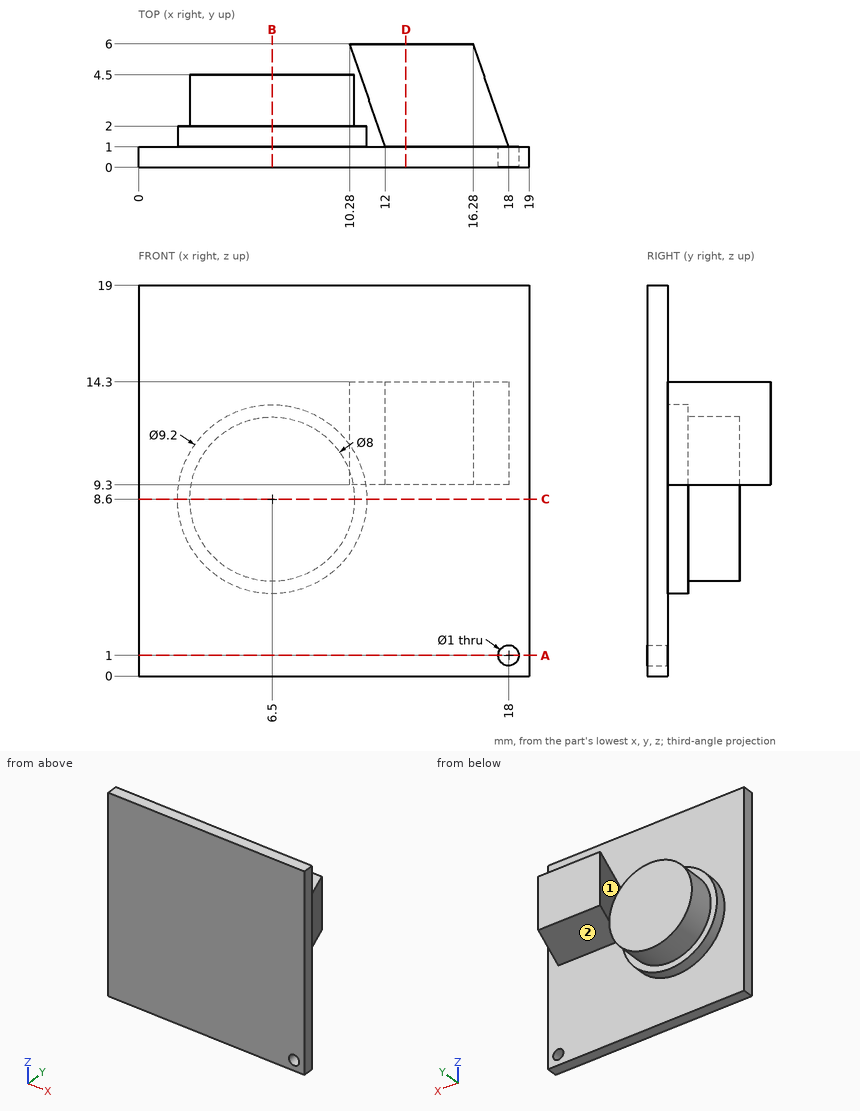
Answer from the drawing. Dimensions are ordinates in mm from the lowest x, y and z of the part. Coordinates: 2 decimals unless noted, no trailing zeros. Write each loop counter-clockwise with the first axis right and the second up, starting at its lowest first coordinate (ties: lowest second). Pieces come first, ordered by that corner, then holes. Notation, with made-up numbers: M 33,-2.75 L 72,-2.75 A10 cw 72,9.25 Z; hole C -28,-32 d11. An arc over 180 degrees is marked long. Use a Markdown table: item, result.
Q1. The part is cut by section D-D, the plane x = 13. Write down the section's boundary in (y, z), then the cut area to 3 significant figures.
Answer block:
| item | result |
|---|---|
| outline | M 0,0 L 1,0 L 1,9.3 L 6,9.3 L 6,14.3 L 1,14.3 L 1,19 L 0,19 Z |
| area | 44.0 mm2 |
Q2. The part is cut by section C-C, the plane z = 8.6. Write down the section's boundary in (x, y), then the cut area to 3 significant figures.
Answer block:
| item | result |
|---|---|
| outline | M 0,0 L 19,0 L 19,1 L 11.1,1 L 11.1,2 L 10.5,2 L 10.5,4.5 L 2.5,4.5 L 2.5,2 L 1.9,2 L 1.9,1 L 0,1 Z |
| area | 48.2 mm2 |
Q3. Determine the mould class of the marked faces 1 and 2 for opening direction X: released by +X, released by -X, zero draft, split by the parting line, or undercut.
Answer block:
| item | result |
|---|---|
| face 1 | undercut |
| face 2 | zero draft |
Q4. Each of these flat-tipped pins is pushed along its axis until it touches: pin 1 Ø1.5 at (x, y) = (15.5, 3.5) entering from +Z; pin 2 Ø1.5 at (x, z) = (13, 8) entering from +Y; pin 3 Ø9.5 at (x, z) = (5.5, 6) entering from +Y; pin 4 Ø1.5 at (x, z) = (7, 12) entering from -Y. Where does it stop, or does it pass through?
Answer block:
| item | result |
|---|---|
| pin 1 | stops at z = 14.3 |
| pin 2 | stops at y = 1 |
| pin 3 | stops at y = 4.5 |
| pin 4 | stops at y = 0 |
Q5. The part is cut by section B-B, the plane x = 6.5. Write down the section's boundary in (y, z), then the cut area to 3 significant figures.
Answer block:
| item | result |
|---|---|
| outline | M 0,0 L 1,0 L 1,4 L 2,4 L 2,4.6 L 4.5,4.6 L 4.5,12.6 L 2,12.6 L 2,13.2 L 1,13.2 L 1,19 L 0,19 Z |
| area | 48.2 mm2 |
Q6. The part is cut by section A-A, the plane z = 1. Write down the section's boundary in (x, y), then the cut area to 3 significant figures.
Answer block:
| item | result |
|---|---|
| outline | M 0,0 L 17.5,0 L 17.5,1 L 0,1 Z; M 18.5,0 L 19,0 L 19,1 L 18.5,1 Z |
| area | 18.0 mm2 |
Q7. Straight lines are drawn through the part: L1, parallel to X at y = 0.7, z = 1; L2, parallel to Z at x = 18, y = 0.75; L3, parallel to Y at x = 11, z = 9. For each, find the intervals that lie inside material, in ascending order. Write a range as [from, to].
Answer block:
| item | result |
|---|---|
| L1 | x = [0, 17.5], [18.5, 19] |
| L2 | z = [0, 0.5], [1.5, 19] |
| L3 | y = [0, 2] |
